Geometry check sheet. Reference: the model listing, model coordinates, mm. A direction names the side the tool comes from. Give positions to 0.01 mm unless a question says otherwise; leave off trailing zeros. Loops run counter-clockwise (first coordinate to the right, second up) from the corner with the lowest first, then second, coordinate; pieces in that order, holes last.
```python
from build123d import *

# Parameters (mm, degrees)
SKETCH1_W             = 10
SKETCH1_H             = 100
BOSS_EXTRUDE1_DEPTH   = 50
SKETCH2_R             = 42
CUT_EXTRUDE1_DEPTH    = 4
CUT_EXTRUDE3_REACH    = 72.965
SKETCH4_R             = 22.75
M3_TAPPED_HOLE1_D     = 2.5
FILLET3_R             = 0.5
CHAMFER1_SIZE         = 1
M4_TAPPED_HOLE1_D     = 3.3
M4_TAPPED_HOLE1_DEPTH = 11
M4_TAPPED_HOLE1_TIP   = 0.991420021
M4_TAPPED_HOLE2_D     = 3.3
M4_TAPPED_HOLE2_DEPTH = 11
M4_TAPPED_HOLE2_TIP   = 0.991420021
M4_TAPPED_HOLE3_D     = 3.3
M4_TAPPED_HOLE3_DEPTH = 11
M4_TAPPED_HOLE3_TIP   = 0.991420021
M4_TAPPED_HOLE4_D     = 3.3
M4_TAPPED_HOLE4_DEPTH = 11
M4_TAPPED_HOLE4_TIP   = 0.991420021
M4_TAPPED_HOLE5_D     = 3.3


with BuildPart() as part:
    # Sketch1 → Boss-Extrude1 (new, symmetric)
    with BuildSketch(Plane(origin=(0, 0, 0), x_dir=(0, 0, -1), z_dir=(1, 0, 0))):
        Rectangle(SKETCH1_W, SKETCH1_H)
    extrude(amount=BOSS_EXTRUDE1_DEPTH, both=True)

    # Sketch2 → Cut-Extrude1 (cut)
    with BuildSketch(Plane.XY.offset(5)):
        Circle(SKETCH2_R)
    extrude(amount=-CUT_EXTRUDE1_DEPTH, mode=Mode.SUBTRACT)

    # Sketch4 → Cut-Extrude3 (cut, up to next)
    with BuildSketch(Plane.XY.offset(1), mode=Mode.PRIVATE) as cut_extrude3_sk1:
        Circle(SKETCH4_R)
    cut_extrude3_tool1 = extrude(cut_extrude3_sk1.sketch, amount=-CUT_EXTRUDE3_REACH, mode=Mode.PRIVATE) & part.part
    add(cut_extrude3_tool1.solids().sort_by_distance((0, 0, 1))[0], mode=Mode.SUBTRACT)

    # M3 Tapped Hole1 (through all)
    with Locations(Plane(origin=(0, 0, -5), x_dir=(1, 0, 0), z_dir=(0, 0, -1))):
        with Locations((35, -12), (-37, 0), (37, 0), (18.5, -32.04293994), (-32.04293994, -18.5), (32.04293994, 18.5), (-18.5, 32.04293994), (0, -37), (0, 37), (-18.5, -32.04293994), (18.5, 32.04293994), (32.04293994, -18.5), (-32.04293994, 18.5), (45, -12)):
            Hole(M3_TAPPED_HOLE1_D / 2)

    # Fillet3
    fillet3_edges = [part.edges().sort_by_distance(p)[0] for p in [
        (-42, 0, 1),
    ]]
    fillet(fillet3_edges, radius=FILLET3_R)

    # Chamfer1
    chamfer1_edges = [part.edges().sort_by_distance(p)[0] for p in [
        (-42, 0, 5),
        (-22.75, 0, 1),
    ]]
    chamfer(chamfer1_edges, length=CHAMFER1_SIZE)

    # M4 Tapped Hole1
    with Locations(Plane(origin=(0, 50, 0), x_dir=(1, 0, 0), z_dir=(0, 1, 0))):
        with Locations((-45, 0), (-25, 0), (25, 0), (45, 0)):
            Hole(M4_TAPPED_HOLE1_D / 2, depth=M4_TAPPED_HOLE1_DEPTH)
            with Locations((0, 0, -(M4_TAPPED_HOLE1_DEPTH + M4_TAPPED_HOLE1_TIP / 2))):  # 118° drill point
                Cone(0, M4_TAPPED_HOLE1_D / 2, M4_TAPPED_HOLE1_TIP, mode=Mode.SUBTRACT)

    # M4 Tapped Hole2
    with Locations(Plane(origin=(0, -50, 0), x_dir=(-1, 0, 0), z_dir=(0, -1, 0))):
        with Locations((45, 0), (25, 0), (-25, 0), (-45, 0)):
            Hole(M4_TAPPED_HOLE2_D / 2, depth=M4_TAPPED_HOLE2_DEPTH)
            with Locations((0, 0, -(M4_TAPPED_HOLE2_DEPTH + M4_TAPPED_HOLE2_TIP / 2))):  # 118° drill point
                Cone(0, M4_TAPPED_HOLE2_D / 2, M4_TAPPED_HOLE2_TIP, mode=Mode.SUBTRACT)

    # M4 Tapped Hole3
    with Locations(Plane(origin=(50, 0, 0), x_dir=(0, 0, -1), z_dir=(1, 0, 0))):
        with Locations((0, 35), (0, -35)):
            Hole(M4_TAPPED_HOLE3_D / 2, depth=M4_TAPPED_HOLE3_DEPTH)
            with Locations((0, 0, -(M4_TAPPED_HOLE3_DEPTH + M4_TAPPED_HOLE3_TIP / 2))):  # 118° drill point
                Cone(0, M4_TAPPED_HOLE3_D / 2, M4_TAPPED_HOLE3_TIP, mode=Mode.SUBTRACT)

    # M4 Tapped Hole4
    with Locations(Plane.ZY.offset(50)):
        with Locations((0, 35), (0, -35)):
            Hole(M4_TAPPED_HOLE4_D / 2, depth=M4_TAPPED_HOLE4_DEPTH)
            with Locations((0, 0, -(M4_TAPPED_HOLE4_DEPTH + M4_TAPPED_HOLE4_TIP / 2))):  # 118° drill point
                Cone(0, M4_TAPPED_HOLE4_D / 2, M4_TAPPED_HOLE4_TIP, mode=Mode.SUBTRACT)

    # M4 Tapped Hole5 (through all)
    with Locations(Plane.XY.offset(5)):
        with Locations((-35.355339059, 35.355339059), (35.355339059, -35.355339059), (35.355339059, 35.355339059), (-35.355339059, -35.355339059)):
            Hole(M4_TAPPED_HOLE5_D / 2)


solid = part.part
```
1) Depth check by flat-ended pin: P1, Ø5.5, axis at x = -45, z = 0, coming from the +Y side; P2, Ø2, axis at x = -25, z = 0, coming from the +Y side; P3, Ø4, axis at x = 32.04, y = 18.5, coming from the +Z side; P4, Ø3, axis at x = -45, z = 0, coming from the +Y side. Enter the tip coordinate at first touch or a pass-through.
2) Mould release check, pull along X, two halves, no side actions. Record for faces 1 (the cylindrical face through (44.42, -33.61, 0.89)), 2 (the conical face through (-38.2, -35.3, 0.1)), 3 (the conical face through (44.714, 38.181, -0.013)): +X half, -X half, draft (parallel to the pull), parting line (faces both ways), or undercut.
3) Scan lines: line 1 along Y through (x, z) = (0, -0.45); line 2 along Y through (x, z) = (19.5, -3); line 3 along Y through (x, z) = (-1, 3.25). Record each from-to range of solid material in increasing order.
4) Sectioned sample at B-B on x = 18.5. Count the separate pieces of the cut face and the enclosed holes in it, plus the area to 3 significant figures.
5) Tool access check on faces 4 (the cylindrical face through (44.42, 36.39, 0.89)), 5 (the cylindrical face through (-44.42, -33.61, -0.89)), 6 (the cylindrical face through (-23.35, 44.42, -0.07)), 7 (the cylindrical face through (-26.65, -44.42, -0.07)). Record the directions out of +Z, -Z, +X, -X, +Y, -Y that give a thin tool (end or side, any length) a straight path to the whole face; none if there is none.
6) Sectioned sample at A-A on y = 0. Enter the section's corners in (x, z).
Determined:
1. P1: stops at y = 50
1. P2: stops at y = 38.61
1. P3: stops at z = 1
1. P4: stops at y = 38.91
2. face 1: draft
2. face 2: -X half
2. face 3: undercut
3. line 1: y = -50 to -38.25, -35.75 to -22.75, 22.75 to 35.75, 38.25 to 50
3. line 2: y = -50 to -32.79, -31.29 to -11.72, 11.72 to 31.29, 32.79 to 50
3. line 3: y = -50 to -41.99, 41.99 to 50
4. separate pieces: 4
4. enclosed holes: 0
4. area: 507 mm2
5. face 4: +X
5. face 5: -X
5. face 6: +Y
5. face 7: -Y
6. outline: (-50, -5) - (-38.25, -5) - (-38.25, 1) - (-41.5, 1) arc R0.5 cw to (-42, 1.5) - (-42, 4) - (-43, 5) - (-50, 5) - close; (-35.75, -5) - (-22.75, -5) - (-22.75, 0) - (-23.75, 1) - (-35.75, 1) - close; (22.75, -5) - (35.75, -5) - (35.75, 1) - (23.75, 1) - (22.75, 0) - close; (38.25, -5) - (50, -5) - (50, 5) - (43, 5) - (42, 4) - (42, 1.5) arc R0.5 cw to (41.5, 1) - (38.25, 1) - close
